Build history of the part. All positions in model axes, mm. Face numbers are marked on the shaded views. A direction names the side the tool comes from. Round coordinates to 2 decimals unless told otherwise and drop trailing zeros. Loops run counter-clockwise (first coordinate to the right, second up) from the corner with the lowest first, then second, coordinate; pieces in that order, holes last. Notation, with made-up numbers: (28.5, -13.75) - (59.5, -13.75) arc R28 ccw to (59.5, 21.25) - close; hole circle Ø11 at (-17.5, 8.5). An arc over 180 degrees is marked (long way). Answer as CSV lines item,"result". Start each with the question number.
```python
from build123d import *

# Parameters (mm, degrees)
SKETCH_W        = 13
SKETCH_H        = 8.2
PAD_DEPTH       = 8.3
SKETCH001_W     = 15.1
SKETCH001_H     = 10.5
PAD001_DEPTH    = 1.4
CHAMFER_SIZE    = 1
PAD002_DEPTH    = 3
FILLET_R        = 1
SKETCH003_W     = 0.33
SKETCH003_H     = 3.7
PAD003_DEPTH    = 6.65
CHAMFER001_SIZE = 1.5
SKETCH004_W     = 1
SKETCH004_H     = 2.5
POCKET_DEPTH    = 11.751


with BuildPart() as part:
    # Sketch → Pad (new body)
    with BuildSketch(Plane.XY):
        Rectangle(SKETCH_W, SKETCH_H)
    extrude(amount=-PAD_DEPTH)

    # Sketch001 → Pad001 (join)
    with BuildSketch(Plane.XY):
        Rectangle(SKETCH001_W, SKETCH001_H)
    extrude(amount=PAD001_DEPTH)

    # Chamfer
    chamfer_edges = [part.edges().sort_by_distance(p)[0] for p in [
        (-7.55, 0, 1.4),
        (0, 5.25, 1.4),
        (7.55, 0, 1.4),
        (0, -5.25, 1.4),
    ]]
    chamfer(chamfer_edges, length=CHAMFER_SIZE)

    # Sketch002 → Pad002 (join, symmetric)
    with BuildSketch(Plane.XZ):
        with BuildLine():
            Line((-5.5, 1.4), (5.5, 1.4))
            ThreePointArc((5.5, 1.4), (4.48879, 3.316002), (2.739315, 4.593869))
            ThreePointArc((-5.5, 1.4), (-1.081654, 2.2264), (2.739315, 4.593869))
        make_face()
    extrude(amount=PAD002_DEPTH, both=True)

    # Fillet
    fillet_edges = [part.edges().sort_by_distance(p)[0] for p in [
        (2.739315, 0, 4.593869),
    ]]
    fillet(fillet_edges, radius=FILLET_R)

    # Sketch003 (on DatumPlane) → Pad003 (join)
    with BuildSketch(Plane.XY.offset(-8.3)):
        with Locations((4.035, 0)):
            Rectangle(SKETCH003_W, SKETCH003_H)
        with Locations((-0.895, 0)):
            Rectangle(SKETCH003_W, SKETCH003_H)
    extrude(amount=-PAD003_DEPTH)

    # Chamfer001
    chamfer001_edges = [part.edges().sort_by_distance(p)[0] for p in [
        (4.035, -1.85, -14.95),
        (4.035, 1.85, -14.95),
        (-0.895, 1.85, -14.95),
        (-0.895, -1.85, -14.95),
    ]]
    chamfer(chamfer001_edges, length=CHAMFER001_SIZE)

    # Sketch004 (on Face5 of Chamfer001) → Pocket (cut, through all)
    with BuildSketch(Plane.YZ.offset(4.2)):
        with Locations((0, -12.51)):
            Rectangle(SKETCH004_W, SKETCH004_H)
    extrude(amount=-POCKET_DEPTH, mode=Mode.SUBTRACT)


solid = part.part
```
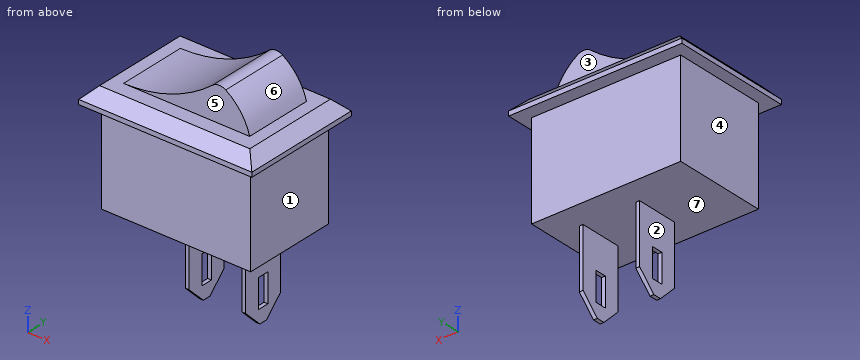
Q1. Wall check: probe 1 along Y at (x, z) = (4.75, -7.5); probe 2 along Y at (x, z) = (0, 1.75); probe 3 along X at (y, z) = (-0.5, -9.5). Give the ranges that are in metal, low to high. Write a range as [from, to].
Q2. Two-plate mould, pull along X, no slides. Class the marked faces 4, 5, 6 and 7: released by +X, released by -X, zero draft, split by the parting line, or undercut.
Q3. Band-saw the part on A-A, the plane z = -11.75. List the corners of the cut face in (x, y), then the cut area to 3 significant figures.
Q4. Pin check, flat tips, straight feed: pin 1 Ø5 at (x, y) = (-2.5, -4) entering from +Z; pin 2 Ø2.5 at (y, z) = (0.5, -2.5) entering from +X; pin 3 Ø1.1 at (y, z) = (0.5, -11.5) entering from +X. Stop position of each tip, or through.
Q5. Tool access for the marked faces 1, 2 and 3: list every direction of +Z, -Z, +X, -X, +Y, -Y with a clear straight run to the whole face (end or side of a thin tool).
Q6. Band-saw the part on C-C, the plane x = -2.5. List the corners of the cut face in (y, z), then the cut area to 3 significant figures.
Q7. Band-saw the part on D-D, the plane z = -2.25. List the corners of the cut face in (x, y), then the cut area to 3 significant figures.
Q8. Band-saw the part on B-B, the plane z = -9.5. List the corners of the cut face in (x, y).
Reported:
1,probe 1,"y = [-4.1, 4.1]"
1,probe 2,"y = [-3, 3]"
1,probe 3,"x = [-1.06, -0.73], [3.87, 4.2]"
2,face 4,"released by -X"
2,face 5,"zero draft"
2,face 6,"released by +X"
2,face 7,"undercut"
3,outline,"(-1.06, -1.85) - (-0.73, -1.85) - (-0.73, -0.5) - (-1.06, -0.5) - close; (-1.06, 0.5) - (-0.73, 0.5) - (-0.73, 1.85) - (-1.06, 1.85) - close; (3.87, -1.85) - (4.2, -1.85) - (4.2, -0.5) - (3.87, -0.5) - close; (3.87, 0.5) - (4.2, 0.5) - (4.2, 1.85) - (3.87, 1.85) - close"
3,area,"1.78 mm2"
4,pin 1,"stops at z = 2.6"
4,pin 2,"stops at x = 6.5"
4,pin 3,"stops at x = 4.2"
5,face 1,"-Z, +X, +Y, -Y"
5,face 2,"-Z, -X, +Y, -Y"
5,face 3,"+Z, +X, -X, +Y"
6,outline,"(-5.25, 0) - (-4.1, 0) - (-4.1, -8.3) - (4.1, -8.3) - (4.1, 0) - (5.25, 0) - (5.25, 0.4) - (4.25, 1.4) - (3, 1.4) - (3, 1.77) - (-3, 1.77) - (-3, 1.4) - (-4.25, 1.4) - (-5.25, 0.4) - close"
6,area,"84.0 mm2"
7,outline,"(-6.5, -4.1) - (6.5, -4.1) - (6.5, 4.1) - (-6.5, 4.1) - close"
7,area,"107 mm2"
8,outline,"(-1.06, -1.85) - (-0.73, -1.85) - (-0.73, 1.85) - (-1.06, 1.85) - close; (3.87, -1.85) - (4.2, -1.85) - (4.2, 1.85) - (3.87, 1.85) - close"
